from build123d import *

# Parameters (mm, degrees)
SKETCH_1_W          = 100
SKETCH_1_H          = 60
EXTRUDE_1_DEPTH     = 48
SKETCH_2_W          = 104
SKETCH_2_H          = 44
CUT_EXTRUDE_1_DEPTH = 40
CUT_EXTRUDE_2_DEPTH = 76.524830354
SKETCH_4_R          = 6
CUT_EXTRUDE_3_DEPTH = 101


with BuildPart() as part:
    # 草图1 → 凸台-拉伸1 (new body)
    with BuildSketch(Plane(origin=(0, 0, 0), x_dir=(1, 0, 0), z_dir=(0, 1, 0))):
        Rectangle(SKETCH_1_W, SKETCH_1_H)
    extrude(amount=EXTRUDE_1_DEPTH)

    # 草图2 → 切除-拉伸1 (cut)
    with BuildSketch(Plane(origin=(0, 48, 0), x_dir=(1, 0, 0), z_dir=(0, 1, 0))):
        Rectangle(SKETCH_2_W, SKETCH_2_H)
    extrude(amount=-CUT_EXTRUDE_1_DEPTH, mode=Mode.SUBTRACT)

    # 草图3 → 切除-拉伸2 (cut, through all)
    with BuildSketch(Plane(origin=(0, 0, 0), x_dir=(1, 0, 0), z_dir=(0, 1, 0))):
        with BuildLine():
            Line((-15, 5), (15, 5))
            ThreePointArc((15, 5), (20, 0), (15, -5))
            Line((15, -5), (-15, -5))
            ThreePointArc((-15, -5), (-20, 0), (-15, 5))
        make_face()
    extrude(amount=CUT_EXTRUDE_2_DEPTH, mode=Mode.SUBTRACT)

    # 草图4 → 切除-拉伸3 (cut, symmetric)
    with BuildSketch(Plane.XY.offset(30)):
        with Locations((-30, 28)):
            Circle(SKETCH_4_R)
        with Locations((30, 28)):
            Circle(SKETCH_4_R)
    extrude(amount=CUT_EXTRUDE_3_DEPTH, both=True, mode=Mode.SUBTRACT)


solid = part.part
Geometry check sheet. Reference: the model listing, model coordinates, mm. A direction names the side the tool comes from. Give positions to 0.01 mm unless a question says otherwise; leave off trailing zeros. Loops run counter-clockwise (first coordinate to the right, second up) from the corner with the lowest first, then second, coordinate; pieces in that order, holes last. Notation, with made-up numbers: (86, 86.25) -> (112, 86.25) arc R31 ccw to (112, 124.25) -> close; hole circle Ø3 at (66.5, 51). An arc over 180 degrees is marked (long way). Answer in a Markdown table with one row per item. Add a question column.
1) Cross-section at C-C on x = 7.5. Record the boundary of the cut face in (y, z).
2) Cross-section at A-A on z = 0. Record the boundary of the cut face in (x, y).
3) Material ranges on probe 1 along Z at (x, y) = (-6.5, 41); probe 2 along Y at (x, z) = (30, 26); probe 3 along Y at (x, z) = (37, -13), recorded low to high. Write a range as from..to.
4) Cross-section at B-B on y = 10.5. Record the boundary of the cut face in (x, z), and give its area (3 significant figures).
5) Cross-section at D-D on y = 28. Record the boundary of the cut face in (x, z).
6) Gauge pin test, flat end, axial feed: P1, Ø7, axis at x = 30, y = 28, coming from the -Z side. Record the tip position at first contact, or that the pin passes through.
7) Set-up check for faces 4 (the face through (-1, 28, -22)), 5 (the face through (-1, 24, -30)), 6 (the face through (0, 4, 5)): record each of +Z, -Z, +X, -X, +Y, -Y from which the full face is reachable in a straight line by a thin tool's end or side.
8) Draft check along Y on faces 1 (the face through (-34.76, 24.35, 26.06)), 2 (the face through (-1, 48, -26)), 3 (the face through (20, 4, 0)). Enter one of: pulls with the +Y half, pulls with the -Y half, needs draft (parallel to the pull), parting line crosses it, or undercut.
Outcome:
| question | item | result |
|---|---|---|
| 1 | outline | (0, -30) -> (48, -30) -> (48, -22) -> (8, -22) -> (8, -5) -> (0, -5) -> close; (0, 5) -> (8, 5) -> (8, 22) -> (48, 22) -> (48, 30) -> (0, 30) -> close |
| 2 | outline | (-50, 0) -> (-20, 0) -> (-20, 8) -> (-50, 8) -> close; (20, 0) -> (50, 0) -> (50, 8) -> (20, 8) -> close |
| 3 | probe 1 | z = -30..-22, 22..30 |
| 3 | probe 2 | y = 0..22, 34..48 |
| 3 | probe 3 | y = 0..8 |
| 4 | outline | (-50, -30) -> (50, -30) -> (50, -22) -> (-50, -22) -> close; (-50, 22) -> (50, 22) -> (50, 30) -> (-50, 30) -> close |
| 4 | area | 1,600 mm^2 |
| 5 | outline | (-50, -30) -> (-36, -30) -> (-36, -22) -> (-50, -22) -> close; (-50, 22) -> (-36, 22) -> (-36, 30) -> (-50, 30) -> close; (-24, -30) -> (24, -30) -> (24, -22) -> (-24, -22) -> close; (-24, 22) -> (24, 22) -> (24, 30) -> (-24, 30) -> close; (36, -30) -> (50, -30) -> (50, -22) -> (36, -22) -> close; (36, 22) -> (50, 22) -> (50, 30) -> (36, 30) -> close |
| 6 | P1 | passes through |
| 7 | face 4 | +X, -X, +Y |
| 7 | face 5 | -Z, +X, -X, +Y, -Y |
| 7 | face 6 | +Y, -Y |
| 8 | face 1 | undercut |
| 8 | face 2 | pulls with the +Y half |
| 8 | face 3 | needs draft |
